The listing builds one solid part. Answer for the finished solid, in the listing's coordinates (mm). Face numbers are marked on the shaded views. A direction names the side the tool comes from. Give positions to 0.01 mm unless a question says otherwise; leave off trailing zeros. Write each loop counter-clockwise with the first axis right and the second up, starting at its lowest first coordinate (ties: lowest second). Pieces come first, ordered by that corner, then holes. Notation, with made-up numbers: (58.25, 89) - (112.25, 89) arc R18 ccw to (112.25, 117) - close; hole circle Ø3 at (-25.5, -32.75). An arc over 180 degrees is marked (long way). Use a Markdown table: item, result. Add a question column.
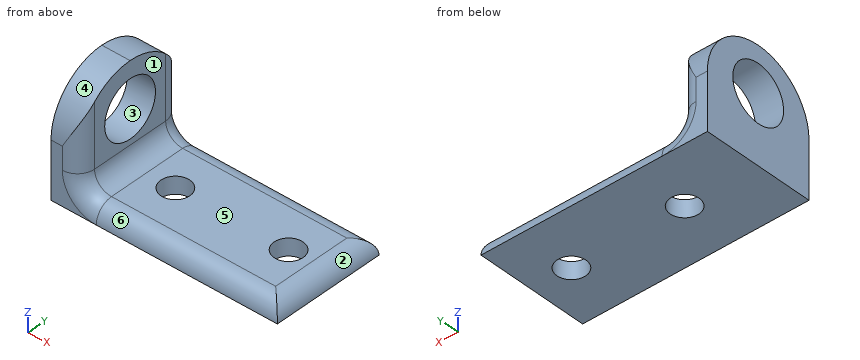
from build123d import *
from OCP.BRepFilletAPI import BRepFilletAPI_MakeFillet

# Parameters (mm, degrees)
SKETCH1_W           = 40
SKETCH1_H           = 20
BOSS_EXTRUDE1_DEPTH = 3
SKETCH2_W           = 5
SKETCH2_H           = 20
BOSS_EXTRUDE2_DEPTH = 20
SKETCH3_R           = 5
CUT_EXTRUDE1_DEPTH  = 31
FILLET2_R           = 10
FILLET2_R_2         = 3
SKETCH4_R           = 2.55
CUT_EXTRUDE2_DEPTH  = 31.000000167


with BuildPart() as part:
    # Sketch1 → Boss-Extrude1 (new body)
    with BuildSketch(Plane.XY):
        Rectangle(SKETCH1_W, SKETCH1_H)
    extrude(amount=BOSS_EXTRUDE1_DEPTH)

    # Sketch2 → Boss-Extrude2 (add)
    with BuildSketch(Plane.XY):
        with Locations((-17.5, 0)):
            Rectangle(SKETCH2_W, SKETCH2_H)
    extrude(amount=BOSS_EXTRUDE2_DEPTH)

    # Sketch3 → Cut-Extrude1 (cut, through all)
    with BuildSketch(Plane(origin=(0, 0, 0), x_dir=(0, 0, -1), z_dir=(1, 0, 0))):
        with Locations((-12, 0)):
            Circle(SKETCH3_R)
    extrude(amount=-CUT_EXTRUDE1_DEPTH, mode=Mode.SUBTRACT)

    # Fillet2
    fillet2_edges_1 = [part.edges().sort_by_distance(p)[0] for p in [
        (-17.5, -10, 20),
        (-17.5, 10, 20),
    ]]
    fillet2_edges_2 = [part.edges().sort_by_distance(p)[0] for p in [
        (2.5, -10, 3),
        (-15, -10, 11.5),
        (-15, 0, 3),
        (-15, 10, 11.5),
        (20, 0, 3),
        (2.5, 10, 3),
    ]]
    fillet2 = BRepFilletAPI_MakeFillet(part.part.solid().wrapped)
    for e in fillet2_edges_1:
        fillet2.Add(FILLET2_R - 0.0001, e.wrapped)
    for e in fillet2_edges_2:
        fillet2.Add(FILLET2_R_2 - 0.0001, e.wrapped)
    add(Compound.cast(fillet2.Shape()), mode=Mode.REPLACE)  # a hair under: the kernel refuses the full size

    # Sketch4 → Cut-Extrude2 (cut, through all)
    with BuildSketch(Plane.XY):
        with Locations(Location((13, 0, 0), (0, 0, 180))):
            Circle(SKETCH4_R)
        with Locations(Location((-7, 0, 0), (0, 0, 180))):
            Circle(SKETCH4_R)
    extrude(amount=CUT_EXTRUDE2_DEPTH, mode=Mode.SUBTRACT)


solid = part.part
1. Given P1, Ø4, axis at x = 6.5, y = -0.5, coming from the +Z side; P2, Ø5, axis at x = 12.5, y = 6, coming from the -Z side; P3, Ø12, axis at y = 5, z = 13, coming from the +X side; P4, Ø11, axis at y = 2, z = 10, coming from the +X side, each flat-ended and moving along its own axis, determine where each tip first touches the part or whether it passes through.
2. Which of the six approach directions +Z, -Z, +X, -X, +Y, -Y give full straight-line access (tool end or side, diameter ignored) to the marked faces 4, 5 and 6?
3. Consider L1, parallel to Z at x = 6.5, y = -1.25; L2, parallel to X at y = 6.25, z = 7; L3, parallel to Y at x = -18.35, z = 12. Determine where each line is inside the solid, lowest interval first. Write a range as [from, to].
4. The part is cut by section C-C (y = -1.25). Count the separate pieces of the cut face and the enclosed holes in it, and give its area (3 significant figures).
5. The part is cut by section B-B (z = 12). Give the vertices of the cut face in (x, y), and give its area (3 significant figures).
6. For a pull along Z with two mould halves and no side action, classify the marked faces 1, 2 and 3 as released by +Z, released by -Z, zero draft, split by the parting line, or undercut.
Check values:
| question | item | result |
|---|---|---|
| 1 | P1 | stops at z = 3 |
| 1 | P2 | stops at z = 0 |
| 1 | P3 | stops at x = -15 |
| 1 | P4 | stops at x = -14.6 |
| 2 | face 4 | +Z, +X, -X, -Y |
| 2 | face 5 | +Z, +X, +Y, -Y |
| 2 | face 6 | +Z, +X, -Y |
| 3 | L1 | z = [0, 3] |
| 3 | L2 | x = [-20, -15] |
| 3 | L3 | y = [-9.8, -5], [5, 9.8] |
| 4 | separate pieces | 4 |
| 4 | enclosed holes | 0 |
| 4 | area | 130 mm2 |
| 5 | outline | (-20, -9.8) - (-16.92, -9.8) arc R3 ccw to (-15, -7) - (-15, -5) - (-20, -5) - close; (-20, 5) - (-15, 5) - (-15, 7) arc R3 ccw to (-16.92, 9.8) - (-20, 9.8) - close |
| 5 | area | 45.0 mm2 |
| 6 | face 1 | zero draft |
| 6 | face 2 | released by +Z |
| 6 | face 3 | undercut |
